CAD build for the part. Positions are in the model's coordinates, mm. Face numbers are marked on the shaded views. A direction names the side the tool comes from. Give positions to 0.01 mm unless a question says otherwise; leave off trailing zeros. Write each loop counter-clockwise with the first axis right and the second up, starting at its lowest first coordinate (ties: lowest second). Pieces come first, ordered by that corner, then holes. Notation, with made-up numbers: (36, 12) -> (61, 12) arc R11 ccw to (61, 19) -> close; hole circle Ø5 at (-35.5, -24). An arc over 180 degrees is marked (long way). Use one line per item in the form item = value. Start each with the question number.
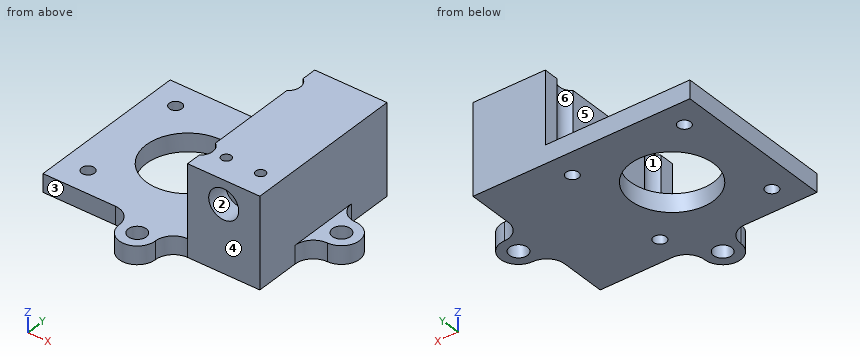
Autodesk Fusion 360 part; units mm, degrees
sketch "Skizze1" plane through (0, 0, 0) normal (0, 0, 1) x (1, 0, 0)
  line L0 (0, 0) -> (60, 0)
  line L1 (60, 0) -> (60, 45)
  line L2 (60, 45) -> (0, 45)
  line L3 (0, 45) -> (0, 0)
  dimension "d1" = 60
  dimension "d2" = 45
extrude "Extrusion1" add sketch "Skizze1" along normal blind 5
sketch "Skizze2" plane through (0, 0, 5) normal (0, 0, 1) x (-1, 0, 0)
  line L0 (0, -45) -> (0, 0)
  line L1 (0, 0) -> (-60, 0)
  line L2 (-60, 0) -> (-60, -45)
  line L3 (-60, -45) -> (0, -45)
  line L4 (0, 0) -> (-45, 0)
  line L5 (-45, 0) -> (-45, -45)
  line L6 (-45, -45) -> (0, -45)
  line L7 (0, -45) -> (0, 0)
  line L8 (-22.5, -45) -> (-22.5, 0)
  line L9 (0, -22.5) -> (-45, -22.5)
  circle A0 centre (-22.5, -22.5) radius 11.5
  line L10 (-22.5, -22.5) -> (-7, -22.5)
  line L11 (-7, -22.5) -> (-7, -38)
  line L12 (-7, -38) -> (-22.5, -38)
  line L13 (-22.5, -38) -> (-22.5, -22.5)
  line L14 (-22.5, -38) -> (-38, -38)
  line L15 (-38, -38) -> (-38, -7)
  line L16 (-7, -22.5) -> (-7, -7)
  line L17 (-38, -7) -> (-7, -7)
  circle A1 centre (-7, -38) radius 1.75
  circle A2 centre (-38, -38) radius 1.75
  circle A3 centre (-38, -7) radius 1.75
  circle A4 centre (-7, -7) radius 1.75
  dimension "d7" = 23
  dimension "d8" = 15.5
  dimension "d9" = 15.5
  dimension "d10" = 31
  dimension "d11" = 3.5
extrude "Extrusion2" cut sketch "Skizze2" against normal blind 5 contours L8 L9 A0 L10 L13 | L8 L9 A0 L10 | L11 L12 A1 | L11 L12 A1 | L16 L17 A4 | L16 L17 A4 | L8 L9 A0 L13 | L14 L15 A2 | L14 L15 A2 | L8 L9 A0 | L15 L17 A3 | L15 L17 A3
sketch "Skizze3" plane through (0, 0, 5) normal (0, 0, 1) x (-1, 0, 0)
  circle A0 centre (-22.5, -22.5) radius 11.5
  circle A1 centre (-38, -38) radius 1.75
  circle A2 centre (-38, -7) radius 1.75
  circle A3 centre (-7, -38) radius 1.75
  circle A4 centre (-7, -7) radius 1.75
  line L0 (0, -45) -> (0, 0)
  line L1 (0, 0) -> (-60, 0)
  line L2 (-60, 0) -> (-60, -45)
  line L3 (-60, -45) -> (0, -45)
  line L4 (-60, 0) -> (-40, 0)
  line L5 (-40, -45) -> (-60, -45)
  line L6 (-60, -45) -> (-60, 0)
  line L7 (-40, -40.8723) -> (-40, -45)
  arc A5 (-40, -35.1277) -> (-40, -40.8723) centre (-38, -38) ccw
  line L8 (-40, 0) -> (-40, -4.1277)
  line L9 (-40, -9.8723) -> (-40, -35.1277)
  arc A6 (-40, -4.1277) -> (-40, -9.8723) centre (-38, -7) ccw
  dimension "d14" = 20
  dimension "d15" = 7
  dimension "d16" = 7
extrude "Extrusion3" add sketch "Skizze3" along normal blind 20 contours L1 L2 L3 L4 L5 L6 L7 A5 L8 L9 A6
sketch "Skizze4" plane through (0, 0, 0) normal (0, 0, -1) x (1, 0, 0)
  circle A0 centre (22.5, -22.5) radius 11.5
  circle A1 centre (38, -38) radius 1.75
  circle A2 centre (38, -7) radius 1.75
  circle A3 centre (7, -38) radius 1.75
  circle A4 centre (7, -7) radius 1.75
  line L0 (0, 0) -> (0, -45)
  line L1 (0, -45) -> (60, -45)
  line L2 (60, -45) -> (60, 0)
  line L3 (60, 0) -> (0, 0)
  line L4 (60, -22.5) -> (70, -22.5)
  line L5 (30, -45) -> (30, -55)
  line L6 (30, -50) -> (40, -50)
  line L7 (40, -50) -> (30, -50)
  line L8 (30, -50) -> (20, -50)
  line L9 (65, -22.5) -> (65, -12.5)
  line L10 (65, -22.5) -> (65, -32.5)
  circle A5 centre (65, -22.5) radius 5
  circle A6 centre (30, -50) radius 5
  circle A7 centre (20, -50) radius 5
  circle A8 centre (40, -50) radius 5
  circle A9 centre (65, -12.5) radius 5
  circle A10 centre (65, -32.5) radius 5
  circle A11 centre (30, -50) radius 2.5
  circle A12 centre (65, -22.5) radius 2.5
  line L11 (30, 0) -> (30, 10)
  line L12 (30, 5) -> (40, 5)
  line L13 (30, 5) -> (20, 5)
  circle A13 centre (30, 5) radius 5
  circle A14 centre (20, 5) radius 5
  circle A15 centre (40, 5) radius 5
  circle A16 centre (30, 5) radius 2.5
  dimension "d19" = 10
  dimension "d20" = 10
  dimension "d21" = 10
  dimension "d22" = 10
  dimension "d27" = 5
  dimension "d28" = 5
  dimension "d35" = 10
  dimension "d36" = 10
  dimension "d37" = 5
extrude "Extrusion4" add sketch "Skizze4" against normal blind 5 contours L3 A13 A14 | L3 A13 A15 | L11 L13 A13 A16 | L11 L12 A13 A16 | L11 L13 A13 A16 | L11 L12 A13 A16 | L2 A5 A9 | L2 A5 A10 | L4 L9 A5 A12 | L4 L10 A5 A12 | L4 L9 A5 A12 | L4 L10 A5 A12
sketch "Skizze5" plane through (0, 45, 0) normal (0, 1, 0) x (-1, 0, 0)
  line L0 (-40, 5) -> (-40, 25)
  line L1 (-40, 25) -> (-60, 25)
  line L2 (-60, 25) -> (-60, 0)
  line L3 (-60, 0) -> (0, 0)
  line L4 (-30, 0) -> (-30, 18.5)
  circle A0 centre (-30, 18.5) radius 4.15
  line L5 (0, 0) -> (0, 5)
  line L6 (0, 5) -> (-40, 5)
  dimension "d31" = 18.5
  dimension "d32" = 8.3
extrude "Extrusion5" cut sketch "Skizze5" against normal blind 6 contours A0
sketch "Skizze6" plane through (0, 0, 0) normal (0, -1, 0) x (1, 0, 0)
  line L0 (40, 5) -> (40, 0)
  line L1 (40, 0) -> (60, 0)
  line L2 (60, 0) -> (60, 25)
  line L3 (60, 25) -> (40, 25)
  line L4 (40, 25) -> (40, 5)
  line L5 (50, 0) -> (50, 18.5)
  circle A0 centre (50, 18.5) radius 4.15
  dimension "d38" = 18.5
  dimension "d39" = 8.3
extrude "Extrusion6" cut sketch "Skizze6" against normal blind 6 contours A0
sketch "Skizze8" plane through (0, 0, 25) normal (0, 0, 1) x (-1, 0, 0)
  line L0 (-40, -4.1277) -> (-40, 0)
  line L1 (-40, 0) -> (-60, 0)
  line L2 (-60, 0) -> (-60, -45)
  line L3 (-60, -45) -> (-40, -45)
  line L4 (-40, -45) -> (-40, -40.8723)
  arc A0 (-40, -35.1277) -> (-40, -40.8723) centre (-38, -38) ccw
  line L5 (-40, -35.1277) -> (-40, -9.8723)
  arc A1 (-40, -4.1277) -> (-40, -9.8723) centre (-38, -7) ccw
  line L6 (-50, 0) -> (-50, -7)
  line L7 (-50, -7) -> (-45.25, -7)
  line L8 (-50, -7) -> (-54.75, -7)
  circle A2 centre (-45.25, -7) radius 1.35
  circle A3 centre (-54.75, -7) radius 1.35
  dimension "d42" = 7
  dimension "d43" = 4.75
  dimension "d44" = 2.7
  dimension "d45" = 2.7
extrude "Extrusion7" cut sketch "Skizze8" against normal blind 5 contours A2 | A3
1) Two-plate mould, pull along Y, no slides. Class the marked faces 4, 5 and 6: released by +Y, released by -Y, zero draft, split by the parting line, or undercut.
2) 3-axis set-ups, long thin cutter, end or side, ignore diameter. For the marked faces 1, 2 and 3: which of +Z, -Z, +X, -X, +Y, -Y reach the whole face in a straight line?
3) Cut at C-C (z = 2.25). Give the cut face in (x, y), and give its area (3 significant figures).
4) Cut at D-D (x = 50). Give the cut face in (y, z), and give its area (3 significant figures).
5) Cut at A-A (y = 22.5). Give the cut face in (x, z), and give its area (3 significant figures).
6) Cut at B-B (x = 38.5). Give the cut face in (y, z), and give its area (3 significant figures).
7) Wall check: line 1 along X through (y, z) = (22.5, 3.55); line 2 along Y through (x, z) = (7, 3.05); line 3 along X through (y, z) = (7, 23.6). Give the ranges that are in metal, low to high. Write a range as from..to.
8) Pin check, flat tips, straight feed: pin 1 (3 mm diameter, centred on x = 25, y = 2.5, fed in from +Z); pin 2 (4.5 mm diameter, centred on y = 44, z = 17, fed in from -X); pin 3 (14 mm diameter, centred on x = 22.5, y = 22.5, fed in from +Z); pin 4 (4 mm diameter, centred on x = 5, z = 2, fed in from -Y). Stop position of each tip, or through.
Final values:
q1.face_4 = released by -Y
q1.face_5 = zero draft
q1.face_6 = undercut
q2.face_1 = +Z, -X
q2.face_2 = -Y
q2.face_3 = +Z, -Z, -X, -Y
q3.outline = (0, 0) -> (20, 0) arc R5 cw to (25, -5) arc R5 ccw to (35, -5) arc R5 cw to (40, 0) -> (60, 0) -> (60, 12.5) arc R5 cw to (65, 17.5) arc R5 ccw to (65, 27.5) arc R5 cw to (60, 32.5) -> (60, 45) -> (0, 45) -> close; hole circle Ø3.5 at (7, 7); hole circle Ø3.5 at (7, 38); hole circle Ø23 at (22.5, 22.5); hole circle Ø5 at (30, -5); hole circle Ø3.5 at (38, 7); hole circle Ø3.5 at (38, 38); hole circle Ø5 at (65, 22.5)
q3.area = 2,410 mm^2
q4.outline = (0, 0) -> (45, 0) -> (45, 25) -> (0, 25) -> (0, 22.65) -> (6, 22.65) -> (6, 14.35) -> (0, 14.35) -> close
q4.area = 1,080 mm^2
q5.outline = (0, 0) -> (11, 0) -> (11, 5) -> (0, 5) -> close; (34, 0) -> (62.5, 0) -> (62.5, 5) -> (60, 5) -> (60, 25) -> (40, 25) -> (40, 5) -> (34, 5) -> close; (67.5, 0) -> (70, 0) -> (70, 5) -> (67.5, 5) -> close
q5.area = 610 mm^2
q6.outline = (-0.23, 0) -> (5.32, 0) -> (5.32, 5) -> (-0.23, 5) -> close; (8.68, 0) -> (36.32, 0) -> (36.32, 5) -> (8.68, 5) -> close; (39.68, 0) -> (45, 0) -> (45, 5) -> (39.68, 5) -> close
q6.area = 193 mm^2
q7.line_1 = 0..11, 34..62.5, 67.5..70
q7.line_2 = 0..5.25, 8.75..36.25, 39.75..45
q7.line_3 = 41.5..43.9, 46.6..53.4, 56.1..60
q8.pin_1 = 5
q8.pin_2 = 40
q8.pin_3 = through
q8.pin_4 = 0
